The model under review builds one solid part; all positions refer to its coordinate system, in mm. A direction names the side the tool comes from. Give positions to 0.01 mm unless a question says otherwise; leave off trailing zeros. Order: outer loops, then holes, each group sorted by start corner. A loop starts at its lowest first (then second) coordinate and runs counter-clockwise, first axis right, second up. Notation, with made-up numbers: (-19, 6) - (40, 6) arc R18 ccw to (40, 16) - close; hole circle Ø10 at (-32, 72). An arc over 180 degrees is marked (long way). Use CSV: the item, a comma, the result in double quotes. Start each with the question number.
1. Machinability: for faces 4 (the conical face through (43.201, 39.458, 6.684)), 5 (the cylindrical face through (41.957, 4.65, 0.651)), 6 (the conical face through (43.347, 39.458, -6.539)), which of the approach directions +Z, -Z, +X, -X, +Y, -Y give a long, thin tool a straight path to every point of the face, cutting with its end or side? Answer none if there is none.
2. To check wall thickness, follow line 1 (Y direction, x = 28, z = 0); line 2 (X direction, y = 6, z = 0); line 3 (Z direction, x = 26.5, y = 76). State the ranges of each line that lie inside material, in increasing order. Write a range as [from, to].
3. For pin 1 (6.5 mm diameter, centred on x = 33, y = 41, fed in from +Z); pin 2 (3 mm diameter, centred on x = 38.5, z = 0, fed in from -Y); pin 3 (4.5 mm diameter, centred on x = 39, z = -3, fed in from +Y); pin 4 (2 mm diameter, centred on x = 39.5, y = 75.5, fed in from -Z), all flat-tipped, find the tip position at first contact; note any pin that passes through.
4. Take a section at B-B, the plane x = 22. State the section outline as (y, z) points, then the cut area to 3 significant figures.
5. Take a section at C-C, the plane y = 76. State the section outline as (x, z) points.
6. Take a section at D-D, the plane y = 62. State the section outline as (x, z) points.
7. Draft analysis for pull direction Y (two halves, no side actions). For faces 1 (the flat face through (30, 34, -10)), 2 (the flat face through (29, -20, 0)), 3 (the conical face through (33.31, 72.71, -0.73)), state which applies: released by +Y, released by -Y, zero draft, split by the parting line, or undercut.
```python
from build123d import *
from OCP.BRepFilletAPI import BRepFilletAPI_MakeChamfer

# Parameters (mm, degrees)
DODANIE_WYCI_GNI_CIE1_DEPTH                        = 100
DODANIE_WYCI_GNI_CIE1_DEPTH_BACK                   = 20
SFAZOWANIE1_SIZE                                   = 10
ZAOKR_GLENIE1_R                                    = 10
SZKIC3_W                                           = 20
SZKIC3_H                                           = 45
WYTNIJ_WYCI_GNI_CIE1_DEPTH                         = 100
SFAZOWANIE2_SIZE                                   = 2
SFAZOWANIE2_SIZE2                                  = 0.890457371
SFAZOWANIE3_SIZE                                   = 2
SFAZOWANIE3_SIZE2                                  = 0.727940469
POG_BIENIE_STO_KOWE_POD_M6_WKR_T_Z_BEM_D           = 6.4
POG_BIENIE_STO_KOWE_POD_M6_WKR_T_Z_BEM_DEPTH       = 40
POG_BIENIE_STO_KOWE_POD_M6_WKR_T_Z_BEM_CSINK_D     = 13.44
POG_BIENIE_STO_KOWE_POD_M6_WKR_T_Z_BEM_CSINK_ANGLE = 90
POG_BIENIE_STO_KOWE_POD_M6_WKR_T_Z_BEM_TIP         = 1.922753981
SZKIC7_R                                           = 5
WYTNIJ_WYCI_GNI_CIE2_DEPTH                         = 50


with BuildPart() as part:
    # Szkic2 → Dodanie-wyciągnięcie1 (new, two sides: drawn at the far end of the back side and taken through both)
    with BuildSketch(Plane(origin=(0, 0, 0), x_dir=(1, 0, 0), z_dir=(0, 1, 0)).offset(-DODANIE_WYCI_GNI_CIE1_DEPTH_BACK)):
        with BuildLine():
            Line((24.162419167, 10), (46.662419167, 10))
            Line((46.662419167, 10), (46.662419167, -10))
            Line((46.662419167, -10), (24.162419167, -10))
            ThreePointArc((24.162419167, -10), (14.53138844, -21.740773905), (0, -26.15))
            Line((0, -26.15), (0, -24.15))
            ThreePointArc((0, -24.15), (24.15, 0), (0, 24.15))
            Line((0, 24.15), (0, 26.15))
            ThreePointArc((0, 26.15), (14.53138844, 21.740773905), (24.162419167, 10))
        make_face()
    extrude(amount=DODANIE_WYCI_GNI_CIE1_DEPTH + DODANIE_WYCI_GNI_CIE1_DEPTH_BACK)

    # Sfazowanie1
    sfazowanie1_edges = [part.edges().sort_by_distance(p)[0] for p in [
        (35.412419167, 100, 10),
        (46.662419167, 100, 0),
        (35.412419167, 100, -10),
    ]]
    chamfer(sfazowanie1_edges, length=SFAZOWANIE1_SIZE - 0.0001)  # a hair under: the kernel refuses the full size

    # Zaokrąglenie1
    zaokr_glenie1_edges = [part.edges().sort_by_distance(p)[0] for p in [
        (46.662419167, 35.00005, -10),
        (46.662419167, 35.00005, 10),
    ]]
    fillet(zaokr_glenie1_edges, radius=ZAOKR_GLENIE1_R - 0.0001)  # a hair under: the kernel refuses the full size

    # Szkic3 → Wytnij-wyciągnięcie1 (cut)
    with BuildSketch(Plane(origin=(36.66, 0, 0), x_dir=(0, 0, -1), z_dir=(1, 0, 0))):
        with Locations((0, 62.5)):
            Rectangle(SZKIC3_W, SZKIC3_H)
    extrude(amount=WYTNIJ_WYCI_GNI_CIE1_DEPTH, mode=Mode.SUBTRACT)

    # Sfazowanie2: one chamfer whose edges measure the first distance from different faces: ONE call of the kernel's chamfer builder (chamfer() names one face for all edges)
    sfazowanie2_edges_1 = [part.edges().sort_by_distance(p)[0] for p in [
        (43.733516268, 40, -7.071097101),
    ]]
    sfazowanie2_side_1 = [part.faces().sort_by_distance(p)[0] for p in [
        (43.733516268, 10, -7.071097101),
    ]]
    sfazowanie2_edges_2 = [part.edges().sort_by_distance(p)[0] for p in [
        (43.733516268, 40, 7.071097101),
    ]]
    sfazowanie2_side_2 = [part.faces().sort_by_distance(p)[0] for p in [
        (43.733516268, 10, 7.071097101),
    ]]
    sfazowanie2_edges_3 = [part.edges().sort_by_distance(p)[0] for p in [
        (36.661259583, 40, -10),
    ]]
    sfazowanie2_side_3 = [part.faces().sort_by_distance(p)[0] for p in [
        (30.411953945, 34.997782587, -10),
    ]]
    sfazowanie2_edges_4 = [part.edges().sort_by_distance(p)[0] for p in [
        (36.661259583, 40, 10),
    ]]
    sfazowanie2_side_4 = [part.faces().sort_by_distance(p)[0] for p in [
        (30.411953945, 34.997782587, 10),
    ]]
    sfazowanie2 = BRepFilletAPI_MakeChamfer(part.part.solid().wrapped)
    for e in sfazowanie2_edges_1:
        sfazowanie2.Add(SFAZOWANIE2_SIZE, SFAZOWANIE2_SIZE2, e.wrapped, sfazowanie2_side_1[0].wrapped)  # the first distance lies on this face
    for e in sfazowanie2_edges_2:
        sfazowanie2.Add(SFAZOWANIE2_SIZE, SFAZOWANIE2_SIZE2, e.wrapped, sfazowanie2_side_2[0].wrapped)  # the first distance lies on this face
    for e in sfazowanie2_edges_3:
        sfazowanie2.Add(SFAZOWANIE2_SIZE, SFAZOWANIE2_SIZE2, e.wrapped, sfazowanie2_side_3[0].wrapped)  # the first distance lies on this face
    for e in sfazowanie2_edges_4:
        sfazowanie2.Add(SFAZOWANIE2_SIZE, SFAZOWANIE2_SIZE2, e.wrapped, sfazowanie2_side_4[0].wrapped)  # the first distance lies on this face
    add(Compound.cast(sfazowanie2.Shape()), mode=Mode.REPLACE)

    # Sfazowanie3: one chamfer whose edges measure the first distance from different faces: ONE call of the kernel's chamfer builder (chamfer() names one face for all edges)
    sfazowanie3_edges_1 = [part.edges().sort_by_distance(p)[0] for p in [
        (43.733516268, 85, -7.071097101),
    ]]
    sfazowanie3_side_1 = [part.faces().sort_by_distance(p)[0] for p in [
        (43.733516268, 88.964501449, -7.071097101),
    ]]
    sfazowanie3_edges_2 = [part.edges().sort_by_distance(p)[0] for p in [
        (43.733516268, 85, 7.071097101),
    ]]
    sfazowanie3_side_2 = [part.faces().sort_by_distance(p)[0] for p in [
        (43.733516268, 88.964501449, 7.071097101),
    ]]
    sfazowanie3_edges_3 = [part.edges().sort_by_distance(p)[0] for p in [
        (36.661259583, 85, -10),
    ]]
    sfazowanie3_side_3 = [part.faces().sort_by_distance(p)[0] for p in [
        (30.411931044, 34.997767921, -10),
    ]]
    sfazowanie3_edges_4 = [part.edges().sort_by_distance(p)[0] for p in [
        (36.661259583, 85, 10),
    ]]
    sfazowanie3_side_4 = [part.faces().sort_by_distance(p)[0] for p in [
        (30.411931044, 34.997767921, 10),
    ]]
    sfazowanie3 = BRepFilletAPI_MakeChamfer(part.part.solid().wrapped)
    for e in sfazowanie3_edges_1:
        sfazowanie3.Add(SFAZOWANIE3_SIZE, SFAZOWANIE3_SIZE2, e.wrapped, sfazowanie3_side_1[0].wrapped)  # the first distance lies on this face
    for e in sfazowanie3_edges_2:
        sfazowanie3.Add(SFAZOWANIE3_SIZE, SFAZOWANIE3_SIZE2, e.wrapped, sfazowanie3_side_2[0].wrapped)  # the first distance lies on this face
    for e in sfazowanie3_edges_3:
        sfazowanie3.Add(SFAZOWANIE3_SIZE, SFAZOWANIE3_SIZE2, e.wrapped, sfazowanie3_side_3[0].wrapped)  # the first distance lies on this face
    for e in sfazowanie3_edges_4:
        sfazowanie3.Add(SFAZOWANIE3_SIZE, SFAZOWANIE3_SIZE2, e.wrapped, sfazowanie3_side_4[0].wrapped)  # the first distance lies on this face
    add(Compound.cast(sfazowanie3.Shape()), mode=Mode.REPLACE)

    # Pogłębienie stożkowe pod M6 Wkręt z łbem stożkowym płaskim2
    with Locations(Plane(origin=(36.66, 0, 0), x_dir=(0, 0, -1), z_dir=(1, 0, 0))):
        with Locations((0, 51), (0, 76)):
            CounterSinkHole(POG_BIENIE_STO_KOWE_POD_M6_WKR_T_Z_BEM_D / 2, POG_BIENIE_STO_KOWE_POD_M6_WKR_T_Z_BEM_CSINK_D / 2, depth=POG_BIENIE_STO_KOWE_POD_M6_WKR_T_Z_BEM_DEPTH, counter_sink_angle=POG_BIENIE_STO_KOWE_POD_M6_WKR_T_Z_BEM_CSINK_ANGLE)
            with Locations((0, 0, -(POG_BIENIE_STO_KOWE_POD_M6_WKR_T_Z_BEM_DEPTH + POG_BIENIE_STO_KOWE_POD_M6_WKR_T_Z_BEM_TIP / 2))):  # 118° drill point
                Cone(0, POG_BIENIE_STO_KOWE_POD_M6_WKR_T_Z_BEM_D / 2, POG_BIENIE_STO_KOWE_POD_M6_WKR_T_Z_BEM_TIP, mode=Mode.SUBTRACT)

    # Szkic7 → Wytnij-wyciągnięcie2 (cut)
    with BuildSketch(Plane.XZ.offset(20)):
        with Locations(Location((37, 0, 0), (0, 0, 270))):
            Circle(SZKIC7_R)
    extrude(amount=-WYTNIJ_WYCI_GNI_CIE2_DEPTH, mode=Mode.SUBTRACT)


solid = part.part
```
Determined:
1,face 4,"+Z, +X"
1,face 5,"-Y"
1,face 6,"-Z, +X"
2,line 1,"y = [-20, 47.8], [54.2, 72.8], [79.2, 100]"
2,line 2,"x = [24.15, 32], [42, 46.66]"
2,line 3,"z = [-10, -3.2], [3.2, 10]"
3,pin 1,"stops at z = 10"
3,pin 2,"stops at y = 30"
3,pin 3,"stops at y = 98.89"
3,pin 4,"passes through"
4,outline,"(-20, -14.14) - (100, -14.14) - (100, -9.96) - (-20, -9.96) - close; (-20, 9.96) - (100, 9.96) - (100, 14.14) - (-20, 14.14) - close"
4,area,"1,000 mm²"
5,outline,"(0, -26.15) arc R26.15 ccw to (24.16, -10) - (36.66, -10) - (36.66, -6.72) - (33.14, -3.2) - (23.94, -3.2) arc R24.15 cw to (0, -24.15) - close; (0, 24.15) arc R24.15 cw to (23.94, 3.2) - (33.14, 3.2) - (36.66, 6.72) - (36.66, 10) - (24.16, 10) arc R26.15 ccw to (0, 26.15) - close"
6,outline,"(0, -26.15) arc R26.15 ccw to (24.16, -10) - (36.66, -10) - (36.66, 10) - (24.16, 10) arc R26.15 ccw to (0, 26.15) - (0, 24.15) arc R24.15 cw to (0, -24.15) - close"
7,face 1,"zero draft"
7,face 2,"released by -Y"
7,face 3,"undercut"
